For this review, take the finished solid that the model builds, in its own axes (mm). Face numbers are marked on the shaded views. A direction names the side the tool comes from. Give positions to 0.01 mm unless a question says otherwise; leave off trailing zeros. Loops run counter-clockwise (first coordinate to the right, second up) from the corner with the lowest first, then second, coordinate; pieces in that order, holes last.
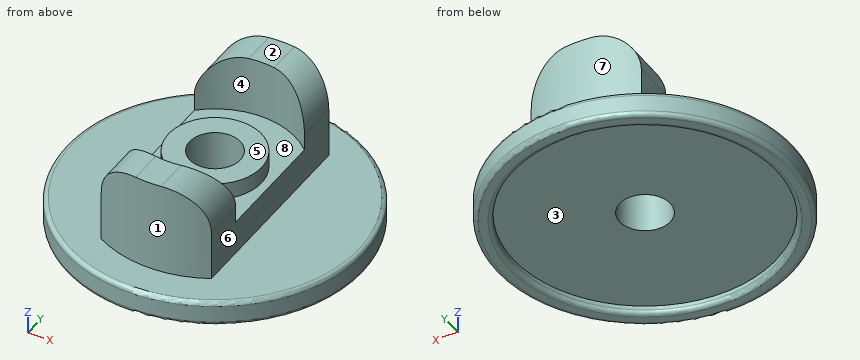
```python
from build123d import *

# Parameters (mm, degrees)
SKETCH1_R           = 17.5
BOSS_EXTRUDE1_DEPTH = 3
SKETCH2_R           = 15.5
CUT_EXTRUDE1_DEPTH  = 1
SKETCH3_W           = 13
SKETCH3_H           = 28
BOSS_EXTRUDE2_DEPTH = 11
SKETCH4_R           = 9.5
CUT_EXTRUDE2_DEPTH  = 7
SKETCH5_R           = 16.54214052
SKETCH5_R_2         = 13.5
CUT_EXTRUDE3_DEPTH  = 11
FILLET1_R           = 5
SKETCH6_R           = 5.5
BOSS_EXTRUDE3_DEPTH = 2
SKETCH7_R           = 3
CUT_EXTRUDE4_DEPTH  = 27.334388165
FILLET3_R           = 0.5


with BuildPart() as part:
    # Sketch1 → Boss-Extrude1 (new body)
    with BuildSketch(Plane.XY):
        Circle(SKETCH1_R)
    extrude(amount=BOSS_EXTRUDE1_DEPTH)

    # Sketch2 → Cut-Extrude1 (cut)
    with BuildSketch(Plane(origin=(0, 0, 0), x_dir=(-1, 0, 0), z_dir=(0, 0, -1))):
        Circle(SKETCH2_R)
    extrude(amount=-CUT_EXTRUDE1_DEPTH, mode=Mode.SUBTRACT)

    # Sketch3 → Boss-Extrude2 (add)
    with BuildSketch(Plane.XY.offset(3)):
        Rectangle(SKETCH3_W, SKETCH3_H)
    extrude(amount=BOSS_EXTRUDE2_DEPTH)

    # Sketch4 → Cut-Extrude2 (cut)
    with BuildSketch(Plane.XY.offset(14)):
        Circle(SKETCH4_R)
    extrude(amount=-CUT_EXTRUDE2_DEPTH, mode=Mode.SUBTRACT)

    # Sketch5 → Cut-Extrude3 (cut)
    with BuildSketch(Plane.XY.offset(14)):
        Circle(SKETCH5_R)
        Circle(SKETCH5_R_2, mode=Mode.SUBTRACT)
    extrude(amount=-CUT_EXTRUDE3_DEPTH, mode=Mode.SUBTRACT)

    # Fillet1
    fillet1_edges = [part.edges().sort_by_distance(p)[0] for p in [
        (6.5, 9.380181398, 14),
        (-6.5, -9.380181398, 14),
        (6.5, -9.380181398, 14),
        (-6.5, 9.380181398, 14),
    ]]
    fillet(fillet1_edges, radius=FILLET1_R)

    # Sketch6 → Boss-Extrude3 (add)
    with BuildSketch(Plane.XY.offset(7)):
        Circle(SKETCH6_R)
    extrude(amount=BOSS_EXTRUDE3_DEPTH)

    # Sketch7 → Cut-Extrude4 (cut, through all)
    with BuildSketch(Plane.XY.offset(9)):
        Circle(SKETCH7_R)
    extrude(amount=-CUT_EXTRUDE4_DEPTH, mode=Mode.SUBTRACT)

    # Fillet3
    fillet3_edges = [part.edges().sort_by_distance(p)[0] for p in [
        (-17.5, 0, 0),
        (-17.5, 0, 3),
        (15.5, 0, 0),
    ]]
    fillet(fillet3_edges, radius=FILLET3_R)


solid = part.part
```
Item 1: Take a section at A-A on y = 0. Give the boundary of the cut face in (x, z), and give its area (3 significant figures).
Answer:
outline: (-17.5, 0.5) arc R0.5 ccw to (-17, 0) - (-16, 0) arc R0.5 ccw to (-15.5, 0.5) - (-15.5, 1) - (-3, 1) - (-3, 9) - (-5.5, 9) - (-5.5, 7) - (-6.5, 7) - (-6.5, 3) - (-17, 3) arc R0.5 ccw to (-17.5, 2.5) - close; (3, 1) - (15.5, 1) - (15.5, 0.5) arc R0.5 ccw to (16, 0) - (17, 0) arc R0.5 ccw to (17.5, 0.5) - (17.5, 2.5) arc R0.5 ccw to (17, 3) - (6.5, 3) - (6.5, 7) - (5.5, 7) - (5.5, 9) - (3, 9) - close
area: 99.7 mm2
Item 2: Take a section at C-C on z = 4.25. Give the boundary of the cut face in (x, y).
Answer:
outline: (-6.5, -11.83) arc R13.5 ccw to (6.5, -11.83) - (6.5, 11.83) arc R13.5 ccw to (-6.5, 11.83) - close; hole circle Ø6 at (0, 0)
Item 3: Tool access review of the marked faces 5, 6, 7 and 8: name each direction out of +Z, -Z, +X, -X, +Y, -Y from which nothing blocks a thin tool from reaching the whole face with its end or side.
Answer:
face 5: +Z, +X, -X
face 6: +Z, +X, +Y, -Y
face 7: +Z, +Y
face 8: +Z
Item 4: Clearance check with flat-ended pins moving along their axes: pin 1 Ø1.8 at (y, z) = (-4.5, 6.5) entering from +X; pin 2 Ø3 at (x, z) = (-11, 2.5) entering from +Y; pin 3 Ø3 at (x, y) = (10, -3) entering from -Z. State where each tip first meets the part, or that it passes through.
Answer:
pin 1: stops at x = 6.5
pin 2: stops at y = 14.7
pin 3: stops at z = 1
Item 5: For L1, parallel to Y at x = 0, z = 0.6; L2, parallel to Z at x = 5, y = 4; L3, parallel to Z at x = 7, y = 9, list the stretches that pass through material, from the lowest coordinate up.
Answer:
L1: y = -17.5 to -15.5, 15.5 to 17.5
L2: z = 1 to 7
L3: z = 1 to 3
Item 6: The part is to be moulded in two halves that separate along X. For the marked faces 1, 2, 3 and 4, say which applies: released by +X, released by -X, zero draft, split by the parting line, or undercut.
Answer:
face 1: split by the parting line
face 2: zero draft
face 3: undercut
face 4: undercut
Item 7: Take a section at D-D on z = 10.25. Give the boundary of the cut face in (x, y), and give its area (3 significant figures).
Answer:
outline: (-6.34, -11.92) arc R13.5 ccw to (6.34, -11.92) - (6.34, -7.07) arc R9.5 cw to (-6.34, -7.07) - close; (-6.34, 7.07) arc R9.5 cw to (6.34, 7.07) - (6.34, 11.92) arc R13.5 ccw to (-6.34, 11.92) - close
area: 108 mm2
